Check sheet for the modelled part. Datum: model origin and axes. Units: mm. A direction names the side the tool comes from. Coordinates: 2 decimals unless noted, no trailing zeros. Loops run counter-clockwise (first coordinate to the right, second up) from the corner with the lowest first, then second, coordinate; pieces in that order, holes last.
```python
from build123d import *

# Parameters (mm, degrees)
F0_W     = 1371.6
F0_H     = 609.6
F1_DEPTH = 25.4
F2_W     = 609.6
F2_H     = 609.6
F3_DEPTH = 25.4
F4_W     = 609.6
F4_H     = 609.6
F5_DEPTH = 25.4
F6_W     = 825.246
F6_H     = 25.4
F7_DEPTH = 609.6
F8_W     = 774.446
F8_H     = 584.2
F9_DEPTH = 12.7


with BuildPart() as f1:
    # F0 (on Top) → F1 (new body)
    with BuildSketch(Plane.XY):
        with Locations((10.840505, -139.387438)):
            Rectangle(F0_W, F0_H)
    extrude(amount=F1_DEPTH)

    # F2 (on face) → F3 (join)
    with BuildSketch(Plane.YZ.offset(696.640505)):
        with Locations((-139.387438, -304.8)):
            Rectangle(F2_W, F2_H)
    extrude(amount=-F3_DEPTH)

    # F4 (on face) → F5 (join)
    with BuildSketch(Plane(origin=(-674.959495, 0, 0), x_dir=(0, -1, 0), z_dir=(-1, 0, 0))):
        with Locations((139.387438, -304.8)):
            Rectangle(F4_W, F4_H)
    extrude(amount=-F5_DEPTH)

    # F6 (on face) → F7 (join)
    with BuildSketch(Plane.XY.offset(25.4)):
        with Locations((284.017505, 152.712562)):
            Rectangle(F6_W, F6_H)
    extrude(amount=F7_DEPTH)

    # F8 (on face) → F9 (cut)
    with BuildSketch(Plane.XZ.offset(-140.012562)):
        with Locations((284.017505, 317.5)):
            Rectangle(F8_W, F8_H)
    extrude(amount=-F9_DEPTH, mode=Mode.SUBTRACT)


solid = f1.part
```
1) Mould release check, pull along X, two halves, no side actions. Record for faces 4 (the flat face through (-297, -444.187, 12)), 5 (the flat face through (279, 152.713, 322)), 6 (the flat face through (-674.959, -135, -288)): +X half, -X half, draft (parallel to the pull), parting line (faces both ways), or undercut.
Answer sheet:
face 4: draft
face 5: undercut
face 6: -X half
2) Section check A-A on z = -410. Enter the section's corners in (x, y).
Answer sheet:
outline: (-674.96, -444.19) - (-649.56, -444.19) - (-649.56, 165.41) - (-674.96, 165.41) - close; (671.24, -444.19) - (696.64, -444.19) - (696.64, 165.41) - (671.24, 165.41) - close
3) Section check B-B on z = 349.5. Enter the section's corners in (x, y).
Answer sheet:
outline: (-128.61, 140.01) - (-103.21, 140.01) - (-103.21, 152.71) - (671.24, 152.71) - (671.24, 140.01) - (696.64, 140.01) - (696.64, 165.41) - (-128.61, 165.41) - close
4) Set-up check for faces 1 (the flat face through (671.241, -144, -301)), 2 (the flat face through (282, 140.013, 622)), 3 (the flat face through (696.641, -144, -273)): record each of +Z, -Z, +X, -X, +Y, -Y from which the full face is reachable in a straight line by a thin tool's end or side.
Answer sheet:
face 1: -Z, +Y, -Y
face 2: +Z, +X, -X, -Y
face 3: +Z, -Z, +X, +Y, -Y
5) Scan lines: line 1 (X direction, y = -101, z = -307); line 2 (Z direction, x = -29, y = -222); line 3 (Y direction, x = -103.5, z = 47). Record each from-to range of solid material in increasing order.
Answer sheet:
line 1: x = -674.96 to -649.56, 671.24 to 696.64
line 2: z = 0 to 25.4
line 3: y = 140.01 to 165.41
6) Section check D-D on x = -574. Enter the section's corners in (y, z), plus the area to 3 significant figures.
Answer sheet:
outline: (-444.19, 0) - (165.41, 0) - (165.41, 25.4) - (-444.19, 25.4) - close
area: 15,500 mm2
7) Depth check by flat-ended pin: pin 1 (20.5 mm diameter, centred on y = 153.5, z = 440.5, fed in from -X); pin 2 (8 mm diameter, centred on x = -111, y = -228, fed in from -Z); pin 3 (4 mm diameter, centred on x = 317.5, y = -172, fed in from +Z). Enter the tip coordinate at first touch or a pass-through.
Answer sheet:
pin 1: stops at x = -128.61
pin 2: stops at z = 0
pin 3: stops at z = 25.4
8) Section check C-C on y = 58. Enter the section's corners in (x, z).
Answer sheet:
outline: (-674.96, -609.6) - (-649.56, -609.6) - (-649.56, 0) - (671.24, 0) - (671.24, -609.6) - (696.64, -609.6) - (696.64, 25.4) - (-674.96, 25.4) - close
